```python
from build123d import *

# Parameters (mm, degrees)
F0_W      = 203.2
F0_H      = 127
F1_DEPTH  = 19.05
F2_R      = 3.048
F3_DEPTH  = 19.051
F4_R      = 3.302
F5_DEPTH  = 12.7
F7_R      = 3.302
F8_DEPTH  = 12.7
F9_R      = 5.461
F10_DEPTH = 3.81


with BuildPart() as f1:
    # F0 (on Front) → F1 (new body)
    with BuildSketch(Plane.XZ):
        Rectangle(F0_W, F0_H)
    extrude(amount=F1_DEPTH)

    # F2 (on face) → F3 (cut, through all)
    with BuildSketch(Plane.XZ.offset(19.05)):
        with Locations((-87.0966, 26.035)):
            Circle(F2_R)
        with Locations((-47.0916, 26.035)):
            Circle(F2_R)
        with Locations((-87.0966, -26.924)):
            Circle(F2_R)
        with Locations((-47.0916, -26.924)):
            Circle(F2_R)
        with Locations((47.0916, -26.924)):
            Circle(F2_R)
        with Locations((47.0916, 26.035)):
            Circle(F2_R)
        with Locations((87.0966, 26.035)):
            Circle(F2_R)
        with Locations((87.0966, -26.924)):
            Circle(F2_R)
    extrude(amount=-F3_DEPTH, mode=Mode.SUBTRACT)

    # F4 (on face) → F5 (cut)
    with BuildSketch(Plane.XY.offset(63.5)):
        with Locations((-76.2, -9.525)):
            Circle(F4_R)
        with Locations((-38.1, -9.525)):
            Circle(F4_R)
        with Locations((0, -9.525)):
            Circle(F4_R)
        with Locations((38.1, -9.525)):
            Circle(F4_R)
        with Locations((76.2, -9.525)):
            Circle(F4_R)
    extrude(amount=-F5_DEPTH, mode=Mode.SUBTRACT)

    # F7 (on face) → F8 (cut)
    with BuildSketch(Plane(origin=(0, 0, -63.5), x_dir=(1, 0, 0), z_dir=(0, 0, -1))):
        with Locations((-76.2, 9.525)):
            Circle(F7_R)
        with Locations((-38.1, 9.525)):
            Circle(F7_R)
        with Locations((0, 9.525)):
            Circle(F7_R)
        with Locations((38.1, 9.525)):
            Circle(F7_R)
        with Locations((76.2, 9.525)):
            Circle(F7_R)
    extrude(amount=-F8_DEPTH, mode=Mode.SUBTRACT)

    # F9 (on face) → F10 (cut)
    with BuildSketch(Plane(origin=(0, 0, 0), x_dir=(-1, 0, 0), z_dir=(0, 1, 0))):
        with Locations((-47.0916, 26.035)):
            Circle(F9_R)
        with Locations((-87.0966, 26.035)):
            Circle(F9_R)
        with Locations((-87.0966, -26.924)):
            Circle(F9_R)
        with Locations((-47.0916, -26.924)):
            Circle(F9_R)
        with Locations((47.0916, -26.924)):
            Circle(F9_R)
        with Locations((87.0966, -26.924)):
            Circle(F9_R)
        with Locations((87.0966, 26.035)):
            Circle(F9_R)
        with Locations((47.0916, 26.035)):
            Circle(F9_R)
    extrude(amount=-F10_DEPTH, mode=Mode.SUBTRACT)


solid = f1.part
```
Verification items for the finished model (mm, model axes). A direction names the side the tool comes from. Give positions to 0.01 mm unless a question says otherwise; leave off trailing zeros. Loops run counter-clockwise (first coordinate to the right, second up) from the corner with the lowest first, then second, coordinate; pieces in that order, holes last.
1. Go/stop test with flat-tipped pins: pin 1 Ø4 at (x, y) = (-76.2, -9.525) entering from -Z; pin 2 Ø3.5 at (x, y) = (77, -9.5) entering from +Z; pin 3 Ø5.5 at (x, z) = (-86.5, 26) entering from +Y. Record where each tip stops, or that it passes through.
2. Mould release check, pull along Z, two halves, no side actions. Record for faces 1 (the flat face through (38, -9, 50.8)), 2 (the cylindrical face through (-73.05, -8.53, 57.24)), 3 (the flat face through (-76, -10, -50.8)), 4 (the flat face through (-49.4, -3.81, 23.7)): released by +Z, released by -Z, zero draft, split by the parting line, or undercut.
3. Set-up check for faces 5 (the cylindrical face through (-92.305, -1.878, -25.284)), 6 (the flat face through (76, -10, -50.8)), 7 (the cylindrical face through (-0.43, -6.25, 57.24)): record each of +Z, -Z, +X, -X, +Y, -Y from which the full face is reachable in a straight line by a thin tool's end or side.
4. Thickness scan on line 1 (Z direction, x = 47.5, y = -5.25); line 2 (Y direction, x = -38, z = 57); line 3 (X direction, y = -12.5, z = -27.5). Record the ranges inside material, lowest first.
5. Section check A-A, the plane x = -76.2. Enter the section's corners in (y, z).
Geometry says:
1. pin 1: stops at z = -50.8
1. pin 2: stops at z = 50.8
1. pin 3: stops at y = -3.81
2. face 1: released by +Z
2. face 2: zero draft
2. face 3: released by -Z
2. face 4: undercut
3. face 5: +Y
3. face 6: -Z
3. face 7: +Z
4. line 1: z = -63.5 to -29.94, -23.9 to 23.01, 29.06 to 63.5
4. line 2: y = -19.05 to -12.83, -6.22 to 0
4. line 3: x = -101.6 to -90.09, -84.1 to -50.08, -44.1 to 44.1, 50.08 to 84.1, 90.09 to 101.6
5. outline: (-19.05, -63.5) - (-12.83, -63.5) - (-12.83, -50.8) - (-6.22, -50.8) - (-6.22, -63.5) - (0, -63.5) - (0, 63.5) - (-6.22, 63.5) - (-6.22, 50.8) - (-12.83, 50.8) - (-12.83, 63.5) - (-19.05, 63.5) - close
